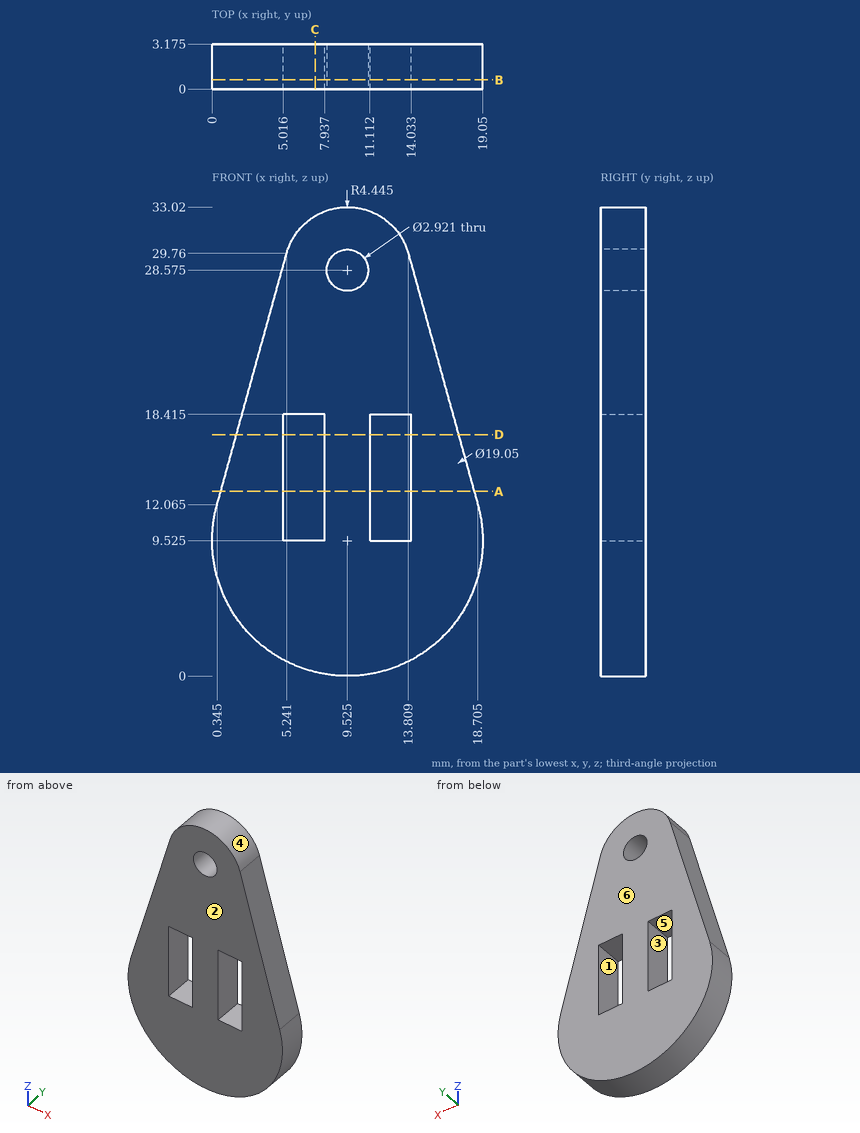
Drawing for the job (mm, zero at the part's lowest x, y, z). A direction names the side the tool comes from. Round coordinates to 2 decimals unless told otherwise and drop trailing zeros. Write each loop counter-clockwise with the first axis right and the second up, starting at its lowest first coordinate (ties: lowest second). Pieces come first, ordered by that corner, then holes. Notation, with made-up numbers: M -1,9 L 24,9 A11 cw 24,21 Z; hole C 57,15 d5. An arc over 180 degrees is marked long. Answer in a Markdown table with one row per item.
1. Saw through at A-A (z = 13). List the corners of the cut face in (x, y) (1 decimal), and give its area (3 significant figures).
Geometry check:
| item | result |
|---|---|
| outline | M 0.6,0 L 5,0 L 5,3.2 L 0.6,3.2 Z; M 7.9,0 L 11.1,0 L 11.1,3.2 L 7.9,3.2 Z; M 14,0 L 18.4,0 L 18.4,3.2 L 14,3.2 Z |
| area | 38.1 mm2 |
2. Probe L1, parallel to X at y = 2, z = 15 (1 decimal); L2, parallel to X at y = 0.5, z = 18 (1 decimal); L3, parallel to Z at x = 9.25, y = 1.4 (1 decimal). List the from-to ranges inside material, lowest first. Write a range as [from, to].
Geometry check:
| item | result |
|---|---|
| L1 | [1.2, 5], [7.9, 11.1], [14, 17.9] |
| L2 | [2, 5], [7.9, 11.1], [14, 17.1] |
| L3 | [0, 27.1], [30, 33] |
3. Saw through at D-D (z = 17). List the corners of the cut face in (x, y) (1 decimal).
Geometry check:
| item | result |
|---|---|
| outline | M 1.7,0 L 5,0 L 5,3.2 L 1.7,3.2 Z; M 7.9,0 L 11.1,0 L 11.1,3.2 L 7.9,3.2 Z; M 14,0 L 17.3,0 L 17.3,3.2 L 14,3.2 Z |
4. Which spindle directions (+Z, -Z, +X, -X, +Y, -Y) get a long thin tool onto all of the face, cutting with end or side? Do the marked faces 1 and 2. Say none if no direction does.
Geometry check:
| item | result |
|---|---|
| face 1 | +Y, -Y |
| face 2 | +Z, -Z, +X, -X, -Y |
5. Mould opens along Z. For the marked faces 3, 4, 5 and 6 say: +Z half, -Z half, draft (parallel to the pull), parting line (faces both ways), or undercut.
Geometry check:
| item | result |
|---|---|
| face 3 | undercut |
| face 4 | +Z half |
| face 5 | undercut |
| face 6 | draft |
6. Saw through at C-C (x = 7.25). List the corners of the cut face in (y, z) (1 decimal).
Geometry check:
| item | result |
|---|---|
| outline | M 0,0.3 L 3.2,0.3 L 3.2,9.5 L 0,9.5 Z; M 0,18.4 L 3.2,18.4 L 3.2,32.4 L 0,32.4 Z |
7. Flat gauge pins, fed straight in: P1, Ø1.5, axis at x = 7.5, y = 0.5, coming from the +Z side; P2, Ø0.9, axis at x = 13, y = 2, coming from the +Z side; P3, Ø1, axis at y = 2, z = 16, coming from the +X side (1 decimal). Where does each tip first touch, or does it go through?
Geometry check:
| item | result |
|---|---|
| P1 | z = 32.83 |
| P2 | z = 31.83 |
| P3 | x = 17.8 |
8. Saw through at B-B (y = 0.65). State how many separate pieces and enclosed holes the cut face has.
Geometry check:
| item | result |
|---|---|
| separate pieces | 1 |
| enclosed holes | 3 |
